Design review of the part built by this model. Coordinates are the model's own, in mm. Coordinates: 2 decimals unless noted, no trailing zeros. Order: outer loops, then holes, each group sorted by start corner. A loop starts at its lowest first (then second) coordinate and runs counter-clockwise, first axis right, second up. Notation, with made-up numbers: M 46,88 L 75,88 A32 cw 75,118 Z; hole C -15.75,74.5 d2. An arc over 180 degrees is marked long. Use CSV: the item, a comma, the result in double quotes.
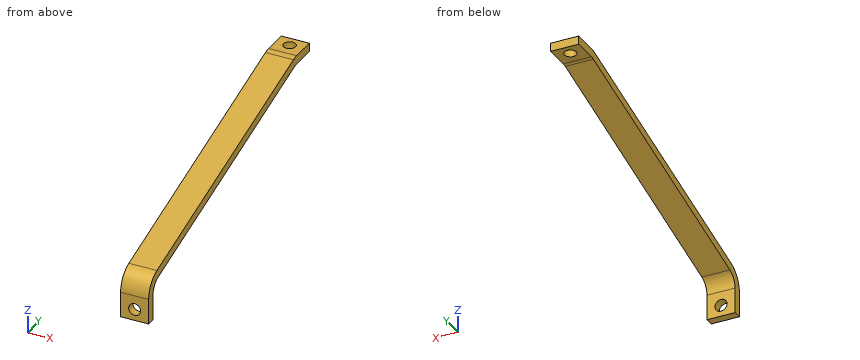
```python
from build123d import *

# Parameters (mm, degrees)
EXTRUDE_1_DEPTH    = 5
HOLE_WIZARD_M4_1_D = 4.3
HOLE_WIZARD_M4_2_D = 4.3


with BuildPart() as part:
    # 草图1 → 拉伸-薄壁1 (new, symmetric)
    with BuildSketch(Plane(origin=(0, 0, 0), x_dir=(0, 0, -1), z_dir=(1, 0, 0))):
        with BuildLine():
            Line((0, 112.09), (0, 103.241097815))
            ThreePointArc((0, 103.241097815), (0.081550018, 102.101734006), (0.324537472, 100.985598982))
            Line((0.324537472, 100.985598982), (28.311930306, 5.744501167))
            ThreePointArc((28.311930306, 5.744501167), (31.193855031, 1.595158446), (35.987392834, 0))
            Line((35.987392834, 0), (45, 0))
            Line((45, 0), (45, 3))
            Line((45, 3), (35.987392834, 3))
            ThreePointArc((35.987392834, 3), (32.991431707, 3.996974029), (31.190228754, 6.59031323))
            Line((31.190228754, 6.59031323), (3.20283592, 101.831411044))
            ThreePointArc((3.20283592, 101.831411044), (3.050968761, 102.528995434), (3, 103.241097815))
            Line((3, 103.241097815), (3, 112.09))
            Line((3, 112.09), (0, 112.09))
        make_face()
    extrude(amount=EXTRUDE_1_DEPTH, both=True)

    # M4 间隙孔1 (through all)
    with Locations(Plane(origin=(0, 0, -3), x_dir=(-1, 0, 0), z_dir=(0, 0, -1))):
        with Locations((0, 108.09)):
            Hole(HOLE_WIZARD_M4_1_D / 2)

    # M4 间隙孔2 (through all)
    with Locations(Plane(origin=(0, 0, 0), x_dir=(-1, 0, 0), z_dir=(0, -1, 0))):
        with Locations((0, 41)):
            Hole(HOLE_WIZARD_M4_2_D / 2)


solid = part.part
```
(1) Add section A-A on x = 0. State the section outline as (y, z) points.
The answers:
outline,"M 0,-45 L 3,-45 L 3,-43.15 L 0,-43.15 Z; M 0,-38.85 L 3,-38.85 L 3,-35.99 A5 cw 6.59,-31.19 L 101.83,-3.2 A5 cw 103.24,-3 L 105.94,-3 L 105.94,0 L 103.24,0 A8 ccw 100.99,-0.32 L 5.74,-28.31 A8 ccw 0,-35.99 Z; M 110.24,-3 L 112.09,-3 L 112.09,0 L 110.24,0 Z"
(2) Add section B-B on y = 108.09. State the section outline as (x, z) points.
The answers:
outline,"M -5,-3 L -2.15,-3 L -2.15,0 L -5,0 Z; M 2.15,-3 L 5,-3 L 5,0 L 2.15,0 Z"
(3) Add section D-D on z = -13.5. State the section outline as (x, y) points, and give its area (3 significant figures).
The answers:
outline,"M -5,56.15 L 5,56.15 L 5,66.79 L -5,66.79 Z"
area,"106 mm2"
(4) Clearance check with flat-ended pins moving along their axes: P1, Ø5, axis at x = 0.5, y = 83.5, coming from the -Z side; P2, Ø3, axis at y = 74.5, z = -5.5, coming from the +X side; P3, Ø4.5, axis at x = 2, z = -41, coming from the +Y side. State where each tip first meets the part, or that it passes through.
The answers:
P1,"stops at z = -9.32"
P2,"passes through"
P3,"stops at y = 3"
(5) Add section C-C on z = -41. State the section outline as (x, y) points.
The answers:
outline,"M -5,0 L -2.15,0 L -2.15,3 L -5,3 Z; M 2.15,0 L 5,0 L 5,3 L 2.15,3 Z"
(6) Wall thickness on probe 1 along X at (y, z) = (1, -41); probe 2 along Z at (x, y) = (0, 1.3); probe 3 along Y at (x, z) = (-2, -38): over which ranges is each line inside the solid? List them lowest first.
The answers:
probe 1,"x = -5 to -2.15, 2.15 to 5"
probe 2,"z = -45 to -43.15, -38.85 to -31.62"
probe 3,"y = 0 to 3"
